Verification items for the finished model (mm, model axes). Face numbers are marked on the shaded views. Give positions to 0.01 mm unless a question says otherwise; leave off trailing zeros. Write each loop counter-clockwise with the first axis right and the second up, starting at its lowest first coordinate (ties: lowest second). Pieces come first, ordered by that corner, then holes. Notation, with made-up numbers: (-0.5, 35) -> (41.5, 35) arc R22 ccw to (41.5, 74) -> close; hole circle Ø9 at (57.5, -34). An arc over 180 degrees is marked (long way). Use one line per item in the form item = value. Start each with the question number.
(1) Release check for a two-part mould opening along Y. For the marked faces 1, 2 and 3 record: pulls with the +Y half, pulls with the -Y half, needs draft (parallel to the pull), parting line crosses it, or undercut.
(2) Section check C-C, the plane x = 7.5. Record the cut outline in (y, z).
(3) Section check A-A, the plane y = 0. Record the cut outline in (x, z).
(4) Scan lines: L1, parallel to Y at x = 3, z = 1; L2, parallel to Z at x = 15.25, y = 0; L3, parallel to Z at x = 12.5, y = 4. Record each from-to range of solid material in increasing order.
from build123d import *

# Parameters (mm, degrees)
F0_W     = 100
F0_H     = 100
F0_R     = 26
F1_DEPTH = 20


with BuildPart() as f1:
    # F0 (on Right) → F1 (new body)
    with BuildSketch(Plane.YZ):
        Rectangle(F0_W, F0_H)
        Circle(F0_R, mode=Mode.SUBTRACT)
    extrude(amount=F1_DEPTH)


solid = f1.part
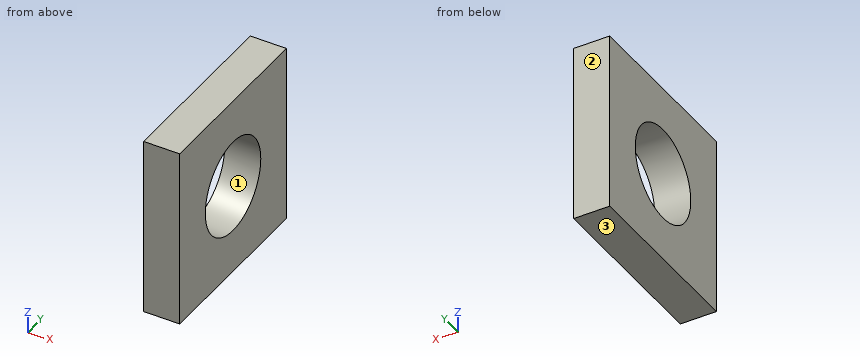
Completed:
q1.face_1 = undercut
q1.face_2 = pulls with the +Y half
q1.face_3 = needs draft
q2.outline = (-50, -50) -> (50, -50) -> (50, 50) -> (-50, 50) -> close; hole circle Ø52 at (0, 0)
q3.outline = (0, -50) -> (20, -50) -> (20, -26) -> (0, -26) -> close; (0, 26) -> (20, 26) -> (20, 50) -> (0, 50) -> close
q4.L1 = -50 to -25.98, 25.98 to 50
q4.L2 = -50 to -26, 26 to 50
q4.L3 = -50 to -25.69, 25.69 to 50
